For this review, use the dimensioned drawing (mm, ordinates from the lowest corner) and the shaded views. Round coordinates to 2 decimals unless told otherwise and drop trailing zeros. Loops run counter-clockwise (first coordinate to the right, second up) from the corner with the lowest first, then second, coordinate; pieces in that order, holes last. Notation, with made-up numbers: M 51.25,57.25 L 71.25,57.25 A14 cw 71.25,75.25 Z; hole C 11,29.5 d6. An arc over 180 degrees is marked long. Answer as a JSON object with one key per item and string values. Group by question number.
Item 1: Consider section B-B (z = 5). Give the boundary of the cut face in (x, y) (1 decimal), and give its area (3 significant figures).
Item 2: Insertion check: P1, Ø4, axis at y = 5.5, z = 6, coming from the -X side; P2, Ø5, axis at x = 15.5, z = 17, coming from the +Y side; P3, Ø1, axis at x = 14.5, z = 17.5, coming from the -Y side. Each pin has a flat end and moves straight along its axis. Give the tip position at first contact, or say it passes through.
Item 3: The part is to be moulded in two halves that separate along X. For the marked faces 1, 2 and 3, say which applies: +X half, -X half, draft (parallel to the pull), parting line (faces both ways), or undercut.
Item 4: To check wall thickness, follow line 1 (Z direction, x = 25, y = 15); line 2 (X direction, y = 24.5, z = 24) (1 decimal); line 3 (Y direction, x = 14, z = 15) (1 decimal). State the ranges of each line that lie inside material, in increasing order.
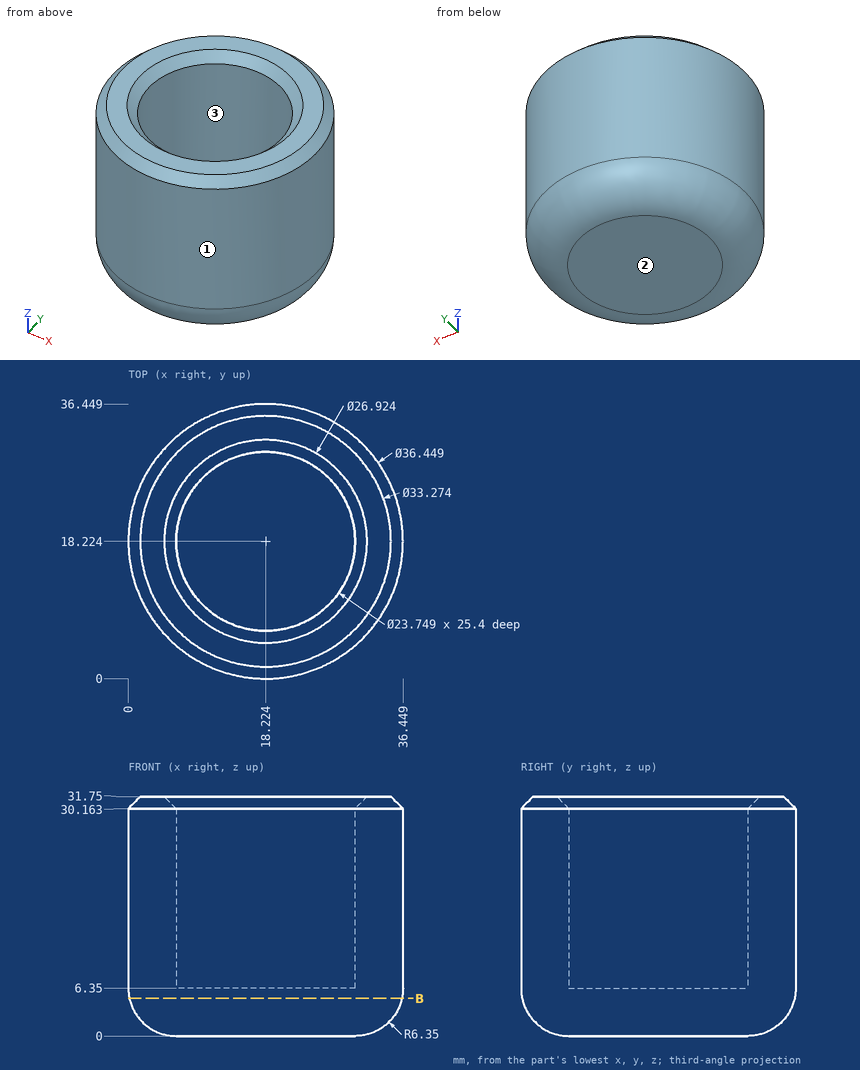
Geometry results:
{
 "1": {"outline": "C 18.2,18.2 d36.2", "area": "1,030 mm^2"},
 "2": {"P1": "stops at x = 3.5", "P2": "stops at y = 36.45", "P3": "stops at y = 0.29"},
 "3": {"face 1": "parting line", "face 2": "draft", "face 3": "undercut"},
 "4": {"line 1": "z = 0 to 6.35", "line 2": "x = 1.1 to 8.1, 28.3 to 35.3", "line 3": "y = 0.5 to 7.1, 29.3 to 36"}
}
